from build123d import *

# Parameters (mm, degrees)
SKETCH_1_W                   = 106
SKETCH_1_H                   = 155
EXTRUDE_1_DEPTH              = 36
SHELL_1_T                    = -2.95
SKETCH_2_W                   = 10
SKETCH_2_H                   = 10
CUT_EXTRUDE_1_DEPTH          = 36
SKETCH_3_W                   = 106
SKETCH_3_H                   = 155
EXTRUDE_2_DEPTH              = 3
HOLE_WIZARD_M4_1_D           = 4.5
HOLE_WIZARD_M4_1_DEPTH       = 45
HOLE_WIZARD_M4_1_CBORE_D     = 8
HOLE_WIZARD_M4_1_CBORE_DEPTH = 4.5
HOLE_WIZARD_M4_1_TIP         = 1.351936393


with BuildPart() as part:
    # 스케치1 → 보스-돌출1 (new body)
    with BuildSketch(Plane.XY):
        Rectangle(SKETCH_1_W, SKETCH_1_H)
    extrude(amount=EXTRUDE_1_DEPTH)

    # 쉘1
    shell_1_openings = [part.faces().sort_by_distance(p)[0] for p in [
        (0, 0, 36),
    ]]
    offset(amount=SHELL_1_T, openings=shell_1_openings, kind=Kind.INTERSECTION)

    # 스케치2 → 컷-돌출1 (cut)
    with BuildSketch(Plane.XZ.offset(77.5)):
        with Locations((0, 8)):
            Rectangle(SKETCH_2_W, SKETCH_2_H)
    extrude(amount=-CUT_EXTRUDE_1_DEPTH, mode=Mode.SUBTRACT)

    # 스케치3 → 보스-돌출2 (add)
    with BuildSketch(Plane(origin=(0, 0, 0), x_dir=(-1, 0, 0), z_dir=(0, 0, -1))):
        Rectangle(SKETCH_3_W, SKETCH_3_H)
    extrude(amount=EXTRUDE_2_DEPTH)

    # M4 소켓 머리 캡 나사용 카운터보어1
    with Locations(Plane.XY.offset(2.95)):
        with Locations((-40, 60), (40, 60), (40, -60), (-40, -60)):
            CounterBoreHole(HOLE_WIZARD_M4_1_D / 2, HOLE_WIZARD_M4_1_CBORE_D / 2, HOLE_WIZARD_M4_1_CBORE_DEPTH, depth=HOLE_WIZARD_M4_1_DEPTH)
            with Locations((0, 0, -(HOLE_WIZARD_M4_1_DEPTH + HOLE_WIZARD_M4_1_TIP / 2))):  # 118° drill point
                Cone(0, HOLE_WIZARD_M4_1_D / 2, HOLE_WIZARD_M4_1_TIP, mode=Mode.SUBTRACT)


solid = part.part
Design review of the part built by this model. Coordinates are the model's own, in mm. A direction names the side the tool comes from. Give positions to 0.01 mm unless a question says otherwise; leave off trailing zeros. Order: outer loops, then holes, each group sorted by start corner. A loop starts at its lowest first (then second) coordinate and runs counter-clockwise, first axis right, second up. Notation, with made-up numbers: (-24, 34) - (33, 34) arc R16 ccw to (33, 42) - close; hole circle Ø9 at (79.5, 35). An arc over 180 degrees is marked (long way). Write item = value, one per line. Start each with the question number.
Q1. To check wall thickness, follow L1, parallel to Y at x = 40, z = -2; L2, parallel to Y at x = 21, z = 25.5; L3, parallel to X at y = 40.5, z = 5.5. State the ranges of each line that lie inside material, in increasing order. Write a range as from..to.
Q2. We need section D-D on x = -1. State the section outline as (y, z) points, plus the area to 3 significant figures.
Q3. Mouldability with a two-part tool opening along Z and no side actions: class faces 1 (the face through (42, -62, -1.55)), 2 (the face through (50.05, -1, 19)), 3 (the face through (0, -76, 13)), 4 (the face through (0, -76, 3)) as released by +Z, released by -Z, zero draft, split by the parting line, or undercut.
Q4. We need section B-B on y = -60. State the section outline as (x, z) points, plus the area to 3 significant figures.
Q5. We need section A-A on x = 40. State the section outline as (y, z) points.
Q6. Tool access review of faces 5 (the face through (-50.05, -1, 19)), 6 (the face through (-5, -76, 8)), 7 (the face through (-38.214, -61.369, -2.285)): name each direction out of +Z, -Z, +X, -X, +Y, -Y from which nothing blocks a thin tool from reaching the whole face with its end or side.
Q7. We need section C-C on z = 15.5. State the section outline as (x, y) points, plus the area to 3 significant figures.
Q8. Clearance check with flat-ended pins moving along their axes: pin 1 Ø3 at (x, y) = (-14.5, -29) entering from +Z; pin 2 Ø4 at (x, y) = (-39, -60) entering from +Z. State where each tip first meets the part, or that it passes through.
Working result:
q1.L1 = -77.5..-62.25, -57.75..57.75, 62.25..77.5
q1.L2 = -77.5..-74.55, 74.55..77.5
q1.L3 = -53..-50.05, 50.05..53
q2.outline = (-77.5, -3) - (77.5, -3) - (77.5, 36) - (74.55, 36) - (74.55, 2.95) - (-74.55, 2.95) - (-74.55, 3) - (-77.5, 3) - close; (-77.5, 13) - (-74.55, 13) - (-74.55, 36) - (-77.5, 36) - close
q2.area = 1,090 mm²
q3.face_1 = released by +Z
q3.face_2 = zero draft
q3.face_3 = undercut
q3.face_4 = undercut
q4.outline = (-53, -3) - (-42.25, -3) - (-42.25, -1.55) - (-44, -1.55) - (-44, 2.95) - (-50.05, 2.95) - (-50.05, 36) - (-53, 36) - close; (-37.75, -3) - (37.75, -3) - (37.75, -1.55) - (36, -1.55) - (36, 2.95) - (-36, 2.95) - (-36, -1.55) - (-37.75, -1.55) - close; (42.25, -3) - (53, -3) - (53, 36) - (50.05, 36) - (50.05, 2.95) - (44, 2.95) - (44, -1.55) - (42.25, -1.55) - close
q4.area = 741 mm²
q5.outline = (-77.5, -3) - (-62.25, -3) - (-62.25, -1.55) - (-64, -1.55) - (-64, 2.95) - (-74.55, 2.95) - (-74.55, 36) - (-77.5, 36) - close; (-57.75, -3) - (57.75, -3) - (57.75, -1.55) - (56, -1.55) - (56, 2.95) - (-56, 2.95) - (-56, -1.55) - (-57.75, -1.55) - close; (62.25, -3) - (77.5, -3) - (77.5, 36) - (74.55, 36) - (74.55, 2.95) - (64, 2.95) - (64, -1.55) - (62.25, -1.55) - close
q6.face_5 = +Z
q6.face_6 = -Y
q6.face_7 = +Z, -Z
q7.outline = (-53, -77.5) - (53, -77.5) - (53, 77.5) - (-53, 77.5) - close; hole (-50.05, -74.55) - (50.05, -74.55) - (50.05, 74.55) - (-50.05, 74.55) - close
q7.area = 1,510 mm²
q8.pin_1 = 2.95
q8.pin_2 = -1.55
